Can you work these out from the model? Positions are in its coordinate system, mm. Coordinates: 2 decimals unless noted, no trailing zeros. Loops run counter-clockwise (first coordinate to the right, second up) from the corner with the lowest first, then second, coordinate; pieces in that order, holes last.
```python
from build123d import *

# Parameters (mm, degrees)
SKETCH1_R           = 2.4
BOSS_EXTRUDE1_DEPTH = 1.8
SKETCH2_R           = 2
BOSS_EXTRUDE2_DEPTH = 2.4
SKETCH3_R           = 2.35
BOSS_EXTRUDE3_DEPTH = 1
CHAMFER1_SIZE       = 0.75
CHAMFER1_SIZE2      = 0.832959386
FILLET1_R           = 0.2
SCALE1_SCALE        = 1.15


with BuildPart() as part:
    # Sketch1 → Boss-Extrude1 (new body)
    with BuildSketch(Plane(origin=(0, 0, 0), x_dir=(1, 0, 0), z_dir=(0, 1, 0))):
        Circle(SKETCH1_R)
    extrude(amount=BOSS_EXTRUDE1_DEPTH)

    # Sketch2 → Boss-Extrude2 (add)
    with BuildSketch(Plane(origin=(0, 1.8, 0), x_dir=(1, 0, 0), z_dir=(0, 1, 0))):
        Circle(SKETCH2_R)
    extrude(amount=BOSS_EXTRUDE2_DEPTH)

    # Sketch3 → Boss-Extrude3 (add)
    with BuildSketch(Plane(origin=(0, 4.2, 0), x_dir=(1, 0, 0), z_dir=(0, 1, 0))):
        Circle(SKETCH3_R)
    extrude(amount=BOSS_EXTRUDE3_DEPTH)

    # Chamfer1
    chamfer1_edges = [part.edges().sort_by_distance(p)[0] for p in [
        (-2.35, 5.2, 0),
    ]]
    chamfer1_side = [part.faces().sort_by_distance(p)[0] for p in [
        (-2.35, 4.7, 0),
    ]]
    chamfer(chamfer1_edges, length=CHAMFER1_SIZE, length2=CHAMFER1_SIZE2, reference=chamfer1_side[0])

    # Fillet1
    fillet1_edges = [part.edges().sort_by_distance(p)[0] for p in [
        (-1.517040614, 5.2, 0),
        (-2.35, 4.45, 0),
        (-2, 1.8, 0),
    ]]
    fillet(fillet1_edges, radius=FILLET1_R)


with BuildPart() as part_1:
    # Scale1: scaled about (-4.5e-08, 2.382820286, 0)
    add(part.part.scale(SCALE1_SCALE).moved(Location((7e-09, -0.357423043, 0))))


solid = part_1.part
```
(1) I want a section at A-A on y = 2.9. Write out the boundary of the cut face in (x, z).
Check values:
outline: circle Ø4.6 at (0, 0)
(2) If I drill on probe 1 along Y at (x, z) = (-0.25, 2.45); probe 2 along Y at (x, z) = (-2.5, 0.6); probe 3 along Z at (x, y) = (0.05, 4), over which ranges is the centre line in solid material (lowest first)?
Check values:
probe 1: y = -0.36 to 1.72, 4.47 to 4.98
probe 2: y = -0.36 to 1.71, 4.47 to 4.88
probe 3: z = -2.3 to 2.3
(3) If we mould it in two halves opening along Y, with no side actions, what happens to faces 1 (the flat face through (0, -0.357, 0)), 2 (the cylindrical face through (-0.598, 0.663, 2.694)), 3 (the cylindrical face through (-2.298, 3.19, -0.101)), 4 (the flat face through (0, 5.623, 0))? For each: released by +Y, released by -Y, zero draft, split by the parting line, or undercut.
Check values:
face 1: released by -Y
face 2: zero draft
face 3: undercut
face 4: released by +Y
(4) I want a section at B-B on y = 0.25. Write out the boundary of the cut face in (x, z), then the cut area to 3 significant figures.
Check values:
outline: circle Ø5.52 at (0, 0)
area: 23.9 mm2
(5) I'm going to push flat-ended pins straight in: pin 1 (1 mm diameter, centred on x = 1.5, y = 2, fed in from +Z); pin 2 (2 mm diameter, centred on x = 1, y = 4.5, fed in from -Z). Where does each tip first touch, or does it pass through?
Check values:
pin 1: stops at z = 2.54
pin 2: stops at z = -2.7
